The listing builds one solid part. Answer for the finished solid, in the listing's coordinates (mm). A direction names the side the tool comes from. Coordinates: 2 decimals unless noted, no trailing zeros. Order: outer loops, then holes, each group sorted by start corner. A loop starts at its lowest first (then second) coordinate and runs counter-clockwise, first axis right, second up. Notation, with made-up numbers: M 57,61.5 L 111,61.5 A11 cw 111,74.5 Z; hole C -36,65 d5. An arc over 180 degrees is marked long. One line per item, written item: value. Start each with the question number.
Q1. For faces 1 (the flat face through (-5.63, -28.28, 52.54)), 2 (the flat face through (-28.28, -5.63, 52.54)), 3 (the cylindrical face through (31.51, 22.07, 52.54)), 4 (the flat face through (-1, -24, 10)), determine the directions among +Z, -Z, +X, -X, +Y, -Y from which every point of the face is accessible in a straight line to the end or side of a thin tool.
Q2. The part is cut by section C-C on y = -31. Give the vertices of the cut face in (x, z).
Q3. Each of these flat-tipped pins is pushed along its axis until it touches: pin 1 Ø9 at (x, y) = (0, 40) entering from -Z; pin 2 Ø6 at (y, z) = (15, 22) entering from +X; pin 3 Ø12 at (x, z) = (-34, 9.5) entering from +Y; pin 4 Ø11.5 at (x, y) = (40, 0) entering from +Z. Where does it stop, or does it pass through?
Q4. The part is cut by section A-A on x = -42. Give the vertices of the cut face in (y, z).
Q5. Straight lines are drawn through the part: line 1 along Y through (x, z) = (0, 11.75); line 2 along Y through (x, z) = (0, 36); line 3 along Y through (x, z) = (1, 7). For each, find the intervals that lie inside material, in ascending order. Write a range as [from, to].
Q6. The part is cut by section D-D on y = 0. Give the vertices of the cut face in (x, z).
Q7. The part is cut by section B-B on z = 21. Give the vertices of the cut face in (x, y).
Q8. Determine the mould class of faces 5 (the flat face through (22, 22, 50)), 6 (the cylindrical face through (36.928, 36.608, 52.535)), 7 (the cylindrical face through (-35, 0, 5)) for opening direction Y: pulls with the +Y half, pulls with the -Y half, needs draft (parallel to the pull), parting line crosses it, or undercut.
```python
from build123d import *

# Parameters (mm, degrees)
SKETCH_R           = 55
SKETCH_R_2         = 9
PAD_DEPTH          = 10
SKETCH001_R        = 5
POCKET_DEPTH       = 321.770145
POLARPATTERN_COUNT = 4
SKETCH002_R        = 21
PAD001_DEPTH       = 45
SKETCH003_R        = 15
POCKET001_DEPTH    = 40
SKETCH004_R        = 9
POCKET002_DEPTH    = 5
SKETCH005_R        = 7
SKETCH005_R_2      = 15
PAD002_DEPTH       = 5


with BuildPart() as part:
    # Sketch → Pad (new body)
    with BuildSketch(Plane.XY):
        Circle(SKETCH_R)
        Circle(SKETCH_R_2, mode=Mode.SUBTRACT)
    extrude(amount=PAD_DEPTH)

    # Sketch001 → Pocket (cut, through all)
    with BuildSketch(Plane.XY.offset(10)):
        with Locations((40, 0)):
            Circle(SKETCH001_R)
    pocket = extrude(amount=-POCKET_DEPTH, mode=Mode.SUBTRACT)

    # PolarPattern: Pocket ×4 about axis
    polarpattern_axis = Axis((0, 0, 10), (0, 0, 1))
    for i in range(1, POLARPATTERN_COUNT):
        add(pocket.rotate(polarpattern_axis, i * 360 / POLARPATTERN_COUNT), mode=Mode.SUBTRACT)

    # Sketch002 → Pad001 (new body)
    with BuildSketch(Plane.XY.offset(10)):
        Circle(SKETCH002_R)
    extrude(amount=PAD001_DEPTH)

    # Sketch003 → Pocket001 (cut)
    with BuildSketch(Plane.XY.offset(55)):
        Circle(SKETCH003_R)
    extrude(amount=-POCKET001_DEPTH, mode=Mode.SUBTRACT)

    # Sketch004 → Pocket002 (cut)
    with BuildSketch(Plane.XY.offset(15)):
        Circle(SKETCH004_R)
    extrude(amount=-POCKET002_DEPTH, mode=Mode.SUBTRACT)

    # Sketch005 → Pad002 (new body)
    with BuildSketch(Plane.XY.offset(55)):
        with BuildLine():
            ThreePointArc((-38.461152, -21.925726), (-36.769553, -36.769553), (-21.925726, -38.461152))
            Line((-21.925726, -38.461152), (11.127411, -17.809568))
            ThreePointArc((11.127411, -17.809568), (14.849242, -14.849243), (17.809568, -11.127412))
            Line((17.809568, -11.127412), (38.461174, 21.925761))
            ThreePointArc((38.461174, 21.925761), (36.769553, 36.769553), (21.925761, 38.461174))
            Line((21.925761, 38.461174), (-11.127412, 17.809568))
            ThreePointArc((-11.127412, 17.809568), (-14.849243, 14.849242), (-17.809568, 11.127411))
            Line((-38.461152, -21.925726), (-17.809568, 11.127411))
        make_face()
        with Locations((-28.284271, -28.284271)):
            Circle(SKETCH005_R, mode=Mode.SUBTRACT)
        with Locations((28.284271, 28.284271)):
            Circle(SKETCH005_R, mode=Mode.SUBTRACT)
        Circle(SKETCH005_R_2, mode=Mode.SUBTRACT)
    extrude(amount=-PAD002_DEPTH)


solid = part.part
```
Output:
1. face 1: +Z, +X, -Y
1. face 2: +Z, -X, +Y
1. face 3: +Z
1. face 4: none
2. outline: M -45.43,0 L 45.43,0 L 45.43,10 L -45.43,10 Z; M -39.97,50 L -34.74,50 L -34.74,55 L -39.97,55 Z; M -21.83,50 L -9.98,50 L -9.98,55 L -21.83,55 Z
3. pin 1: passes through
3. pin 2: stops at x = 17.23
3. pin 3: stops at y = 47.34
3. pin 4: stops at z = 10
4. outline: M -35.51,0 L -4.58,0 L -4.58,10 L -35.51,10 Z; M 4.58,0 L 35.51,0 L 35.51,10 L 4.58,10 Z
5. line 1: y = [-21, -9], [9, 21]
5. line 2: y = [-21, -15], [15, 21]
5. line 3: y = [-54.99, -44.9], [-35.1, -8.94], [8.94, 35.1], [44.9, 54.99]
6. outline: M -55,0 L -45,0 L -45,10 L -55,10 Z; M -35,0 L -9,0 L -9,15 L -15,15 L -15,55 L -24.76,55 L -24.76,50 L -21,50 L -21,10 L -35,10 Z; M 9,0 L 35,0 L 35,10 L 21,10 L 21,50 L 24.76,50 L 24.76,55 L 15,55 L 15,15 L 9,15 Z; M 45,0 L 55,0 L 55,10 L 45,10 Z
7. outline: C 0,0 d42; hole C 0,0 d30
8. face 5: needs draft
8. face 6: parting line crosses it
8. face 7: undercut
